from build123d import *

# Parameters (mm, degrees)
SKETCH1_R           = 42.8625
SKETCH1_R_2         = 2.15
BOSS_EXTRUDE1_DEPTH = 2.54
CUT_EXTRUDE1_START  = -2.54
CUT_EXTRUDE1_DEPTH  = 2.54
SKETCH6_R           = 4.7625
SKETCH6_R_2         = 2.15
BOSS_EXTRUDE4_DEPTH = 12.7


with BuildPart() as part:
    # Sketch1 → Boss-Extrude1 (new body)
    with BuildSketch(Plane(origin=(0, 0, 0), x_dir=(1, 0, 0), z_dir=(0, 1, 0))):
        with Locations(Location((0, 0, 0), (0, 0, 270))):
            Circle(SKETCH1_R)
        with Locations(Location((0, 38.1, 0), (0, 0, 270))):
            Circle(SKETCH1_R_2, mode=Mode.SUBTRACT)
        with Locations(Location((32.995567884, -19.05, 0), (0, 0, 270))):
            Circle(SKETCH1_R_2, mode=Mode.SUBTRACT)
        with Locations(Location((-32.995567884, -19.05, 0), (0, 0, 270))):
            Circle(SKETCH1_R_2, mode=Mode.SUBTRACT)
    extrude(amount=BOSS_EXTRUDE1_DEPTH)

    # Sketch2 → Cut-Extrude1 (cut)
    with BuildSketch(Plane(origin=(0, 2.54, 0), x_dir=(1, 0, 0), z_dir=(0, 1, 0)).offset(CUT_EXTRUDE1_START)):
        with BuildLine():
            Line((-37.12001387, -16.66875), (-4.124445986, 40.48125))
            ThreePointArc((-4.124445986, 40.48125), (-2.381249978, 42.224445998), (5.1e-08, 42.8625))
            ThreePointArc((5.1e-08, 42.8625), (-37.120013889, 21.431249967), (-37.120013806, -21.431250111))
            ThreePointArc((-37.120013806, -21.431250111), (-37.758067884, -19.050000064), (-37.12001387, -16.66875))
        make_face()
        with BuildLine():
            ThreePointArc((37.120013869, -21.431250002), (37.120013883, 21.431249977), (5.1e-08, 42.8625))
            ThreePointArc((5.1e-08, 42.8625), (2.381250022, 42.224445973), (4.124445986, 40.48125))
            Line((4.124445986, 40.48125), (37.12001387, -16.66875))
            ThreePointArc((37.12001387, -16.66875), (37.758067884, -19.050000001), (37.120013869, -21.431250002))
        make_face()
        with BuildLine():
            ThreePointArc((-32.995567884, -23.8125), (-35.376817829, -23.174446018), (-37.120013806, -21.431250111))
            ThreePointArc((-37.120013806, -21.431250111), (6.3e-08, -42.8625), (37.120013869, -21.431250002))
            ThreePointArc((37.120013869, -21.431250002), (35.376817883, -23.174445986), (32.995567884, -23.8125))
            Line((32.995567884, -23.8125), (-32.995567884, -23.8125))
        make_face()
    extrude(amount=CUT_EXTRUDE1_DEPTH, mode=Mode.SUBTRACT)

    # Sketch6 → Boss-Extrude4 (add)
    # profile 1 of 3: a face of its own
    with BuildSketch(Plane(origin=(0, 2.54, 0), x_dir=(1, 0, 0), z_dir=(0, 1, 0))):
        with Locations(Location((0, 38.1, 0), (0, 0, 270))):
            Circle(SKETCH6_R)
        with Locations(Location((0, 38.1, 0), (0, 0, 270))):
            Circle(SKETCH6_R_2, mode=Mode.SUBTRACT)
    # profile 2 of 3: a face of its own
    with BuildSketch(Plane(origin=(0, 2.54, 0), x_dir=(1, 0, 0), z_dir=(0, 1, 0))):
        with Locations(Location((32.995567884, -19.05, 0), (0, 0, 270))):
            Circle(SKETCH6_R)
        with Locations(Location((32.995567884, -19.05, 0), (0, 0, 270))):
            Circle(SKETCH6_R_2, mode=Mode.SUBTRACT)
    # profile 3 of 3: a face of its own
    with BuildSketch(Plane(origin=(0, 2.54, 0), x_dir=(1, 0, 0), z_dir=(0, 1, 0))):
        with Locations(Location((-32.995567884, -19.05, 0), (0, 0, 270))):
            Circle(SKETCH6_R)
        with Locations(Location((-32.995567884, -19.05, 0), (0, 0, 270))):
            Circle(SKETCH6_R_2, mode=Mode.SUBTRACT)
    extrude(amount=BOSS_EXTRUDE4_DEPTH)


solid = part.part
Read the model definition and answer for the solid it produces. Units are mm, in the model's axes. Coordinates: 2 decimals unless noted, no trailing zeros. Loops run counter-clockwise (first coordinate to the right, second up) from the corner with the lowest first, then second, coordinate; pieces in that order, holes last. Notation, with made-up numbers: (21.25, 7) - (69.25, 7) arc R15 cw to (69.25, 25) - close; hole circle Ø5 at (-5.5, -32). An arc over 180 degrees is marked (long way). Answer in a Markdown table with one row per item.
Q1. Find section D-D on z = -17.5. Write down the section's boundary in (x, y).
Here are the results:
| item | result |
|---|---|
| outline | (-17.39, 0) - (17.39, 0) - (17.39, 2.54) - (-17.39, 2.54) - close |
Q2. Find section B-B on z = 19.05. Write down the section's boundary in (x, y), plus the area to 3 significant figures.
Here are the results:
| item | result |
|---|---|
| outline | (-37.76, 0) - (-35.15, 0) - (-35.15, 15.24) - (-37.76, 15.24) - close; (-30.85, 0) - (30.85, 0) - (30.85, 15.24) - (28.23, 15.24) - (28.23, 2.54) - (-28.23, 2.54) - (-28.23, 15.24) - (-30.85, 15.24) - close; (35.15, 0) - (37.76, 0) - (37.76, 15.24) - (35.15, 15.24) - close |
| area | 303 mm^2 |
Q3. Given P1, Ø5, axis at y = 6.5, z = -9, coming from the -X side; P2, Ø6, axis at y = 12, z = 14.5, coming from the +X side, each flat-ended and moving along its own axis, determine where each tip first touches the part or whether it passes through.
Here are the results:
| item | result |
|---|---|
| P1 | passes through |
| P2 | stops at x = 37.5 |
Q4. Find section C-C on z = -37. Write down the section's boundary in (x, y).
Here are the results:
| item | result |
|---|---|
| outline | (-6.13, 0) - (-1.85, 0) - (-1.85, 15.24) - (-4.63, 15.24) - (-4.63, 2.54) - (-6.13, 2.54) - close; (1.85, 0) - (6.13, 0) - (6.13, 2.54) - (4.63, 2.54) - (4.63, 15.24) - (1.85, 15.24) - close |
Q5. Find section A-A on y = 12.75. Count the separate pieces of the cut face and the enclosed holes in it, plus the area to 3 significant figures.
Here are the results:
| item | result |
|---|---|
| separate pieces | 3 |
| enclosed holes | 3 |
| area | 170 mm^2 |
Q6. Straight lines are drawn through the part: line 1 along X through (y, z) = (9, 19.05); line 2 along X through (y, z) = (14.75, 20.5); line 3 along Y through (x, z) = (12, -17). For each, find the intervals that lie inside material, in ascending order. Write a range as [from, to].
Here are the results:
| item | result |
|---|---|
| line 1 | x = [-37.76, -35.15], [-30.85, -28.23], [28.23, 30.85], [35.15, 37.76] |
| line 2 | x = [-37.53, -34.58], [-31.41, -28.46], [28.46, 31.41], [34.58, 37.53] |
| line 3 | y = [0, 2.54] |
Q7. The mould has two halves that part along X. Classify faces 1 (the flat face through (-31.9, 15.24, 21.1)), 2 (the cylindrical face through (31.69, 7.51, 17.34)), 3 (the flat face through (-20.85, 1.25, -11.51)): pulls with the +X half, pulls with the -X half, needs draft (parallel to the pull), parting line crosses it, or undercut.
Here are the results:
| item | result |
|---|---|
| face 1 | needs draft |
| face 2 | undercut |
| face 3 | pulls with the -X half |
